Geometry check sheet. Reference: drawing and pictorial views, mm from the part's lowest x, y, z. Coordinates: 2 decimals unless noted, no trailing zeros. Write each loop counter-clockwise with the first axis right and the second up, starting at its lowest first coordinate (ties: lowest second). Pieces come first, ordered by that corner, then holes.
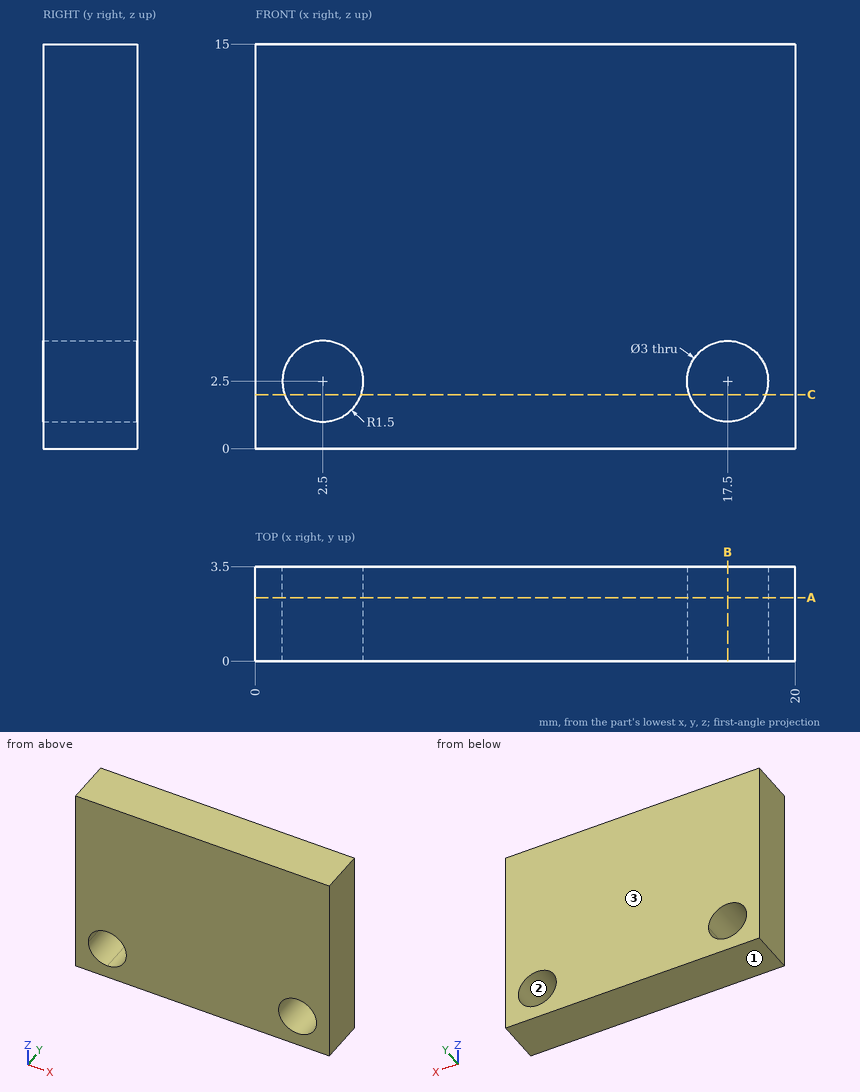
1. Material ranges on L1, parallel to X at y = 1.4, z = 2.5; L2, parallel to X at y = 2, z = 3; L3, parallel to Z at x = 1.25, y = 1.45, recorded low to high.
2. Gauge pin test, flat end, axial feed: P1, Ø2, axis at x = 5, y = 0.5, coming from the -Z side. Record the tip position at first contact, or that the pin passes through.
3. Draft check along Z on the marked faces 1, 2 and 3. Enter one of: pulls with the +Z half, pulls with the -Z half, needs draft (parallel to the pull), parting line crosses it, or undercut.
4. Sectioned sample at C-C, the plane z = 2. Record the boundary of the cut face in (x, y), and give its area (3 significant figures).
5. Sectioned sample at B-B, the plane x = 17.5. Record the boundary of the cut face in (y, z), and give its area (3 significant figures).
6. Sectioned sample at A-A, the plane y = 2.35. Record the boundary of the cut face in (x, z).
Outcome:
1. L1: x = 0 to 1, 4 to 16, 19 to 20
1. L2: x = 0 to 1.09, 3.91 to 16.09, 18.91 to 20
1. L3: z = 0 to 1.67, 3.33 to 15
2. P1: stops at z = 0
3. face 1: pulls with the -Z half
3. face 2: undercut
3. face 3: needs draft
4. outline: (0, 0) - (1.09, 0) - (1.09, 3.5) - (0, 3.5) - close; (3.91, 0) - (16.09, 0) - (16.09, 3.5) - (3.91, 3.5) - close; (18.91, 0) - (20, 0) - (20, 3.5) - (18.91, 3.5) - close
4. area: 50.2 mm2
5. outline: (0, 0) - (3.5, 0) - (3.5, 1) - (0, 1) - close; (0, 4) - (3.5, 4) - (3.5, 15) - (0, 15) - close
5. area: 42.0 mm2
6. outline: (0, 0) - (20, 0) - (20, 15) - (0, 15) - close; hole circle Ø3 at (2.5, 2.5); hole circle Ø3 at (17.5, 2.5)
